```python
from build123d import *

# Parameters (mm, degrees)
SKETCH1_R           = 14.2875
SKETCH1_R_2         = 9.5885
SKETCH1_R_3         = 3.175
SKETCH1_R_4         = 2.257278931
SKETCH1_R_5         = 2.521989484
SKETCH1_R_6         = 2.481468777
SKETCH1_R_7         = 3.567111366
BOSS_EXTRUDE1_DEPTH = 3.175
FILLET1_R           = 9.525
FILLET2_R           = 3.175
FILLET3_R           = 6.35


with BuildPart() as part:
    # Sketch1 → Boss-Extrude1 (new, symmetric)
    with BuildSketch(Plane.XY):
        with BuildLine():
            Line((-35.563882813, 47.798897166), (35.563882813, 47.798897166))
            Line((35.563882813, 47.798897166), (51.692882813, 47.798897166))
            Line((51.692882813, 47.798897166), (67.821882813, 31.669897166))
            Line((67.821882813, 31.669897166), (67.821882813, 15.540897166))
            ThreePointArc((67.821882813, 15.540897166), (62.208310766, -2.642969943), (47.321354383, -14.498084612))
            Line((47.321354383, -14.498084612), (7.26457678, -33.02))
            Line((7.26457678, -33.02), (-7.26457678, -33.02))
            Line((-7.26457678, -33.02), (-47.321354383, -14.498084612))
            ThreePointArc((-47.321354383, -14.498084612), (-62.208310766, -2.642969943), (-67.821882813, 15.540897166))
            Line((-67.821882813, 15.540897166), (-67.821882813, 31.669897166))
            Line((-67.821882813, 31.669897166), (-51.692882813, 47.798897166))
            Line((-51.692882813, 47.798897166), (-35.563882813, 47.798897166))
        make_face()
        Circle(SKETCH1_R, mode=Mode.SUBTRACT)
        with Locations((35.563882813, 15.540897166)):
            Circle(SKETCH1_R_2, mode=Mode.SUBTRACT)
        with Locations((-35.563882813, 15.540897166)):
            Circle(SKETCH1_R_2, mode=Mode.SUBTRACT)
        with Locations((-47.625, 0)):
            Circle(SKETCH1_R_3, mode=Mode.SUBTRACT)
        with Locations((47.625, 0)):
            Circle(SKETCH1_R_3, mode=Mode.SUBTRACT)
        with Locations((-35.563882813, 40.940897166)):
            Circle(SKETCH1_R_4, mode=Mode.SUBTRACT)
        with Locations((-35.563882813, -9.859102834)):
            Circle(SKETCH1_R_5, mode=Mode.SUBTRACT)
        with Locations((35.563882813, -9.859102834)):
            Circle(SKETCH1_R_6, mode=Mode.SUBTRACT)
        with Locations((35.563882813, 40.940897166)):
            Circle(SKETCH1_R_7, mode=Mode.SUBTRACT)
    extrude(amount=BOSS_EXTRUDE1_DEPTH, both=True)

    # Fillet1
    fillet1_edges = [part.edges().sort_by_distance(p)[0] for p in [
        (51.692882813, 47.798897166, 0),
        (-51.692882813, 47.798897166, 0),
    ]]
    fillet(fillet1_edges, radius=FILLET1_R)

    # Fillet2
    fillet2_edges = [part.edges().sort_by_distance(p)[0] for p in [
        (67.821882813, 31.669897166, 0),
        (-67.821882813, 31.669897166, 0),
    ]]
    fillet(fillet2_edges, radius=FILLET2_R)

    # Fillet3
    fillet3_edges = [part.edges().sort_by_distance(p)[0] for p in [
        (7.26457678, -33.02, 0),
        (-7.26457678, -33.02, 0),
    ]]
    fillet(fillet3_edges, radius=FILLET3_R)


solid = part.part
```
For this review, take the finished solid that the model builds, in its own axes (mm). Coordinates: 2 decimals unless noted, no trailing zeros. Order: outer loops, then holes, each group sorted by start corner. A loop starts at its lowest first (then second) coordinate and runs counter-clockwise, first axis right, second up. Notation, with made-up numbers: (55, 89.25) -> (100, 89.25) arc R23 cw to (100, 107.25) -> close; hole circle Ø2 at (-36, 16). An arc over 180 degrees is marked (long way). Use CSV: the item, a comma, the result in double quotes. Start each with the question number.
Item 1: Insertion check: pin 1 (4 mm diameter, centred on x = -35.56, y = 40.94, fed in from +Z); pin 2 (1 mm diameter, centred on x = -30.5, z = 1, fed in from -Y); pin 3 (2 mm diameter, centred on y = 6, z = 1.5, fed in from +X). Each pin has a flat end and moves straight along its axis. Give the tip position at first contact, or say it passes through.
Item 2: We need section B-B, the plane y = 22. Give the boundary of the cut face in (x, z) (3 decimals), then the cut area to 3 significant figures.
Item 3: Draft analysis for pull direction X (two halves, no side actions). For faces 1 (the face through (1, 17, 3.175)), 2 (the face through (67.822, 23, 0)), 3 (the face through (-44.597, 0.954, -0.044)), 4 (the face through (-37.42, -8.15, -0.04)), state which applies: pulls with the +X half, pulls with the -X half, needs draft (parallel to the pull), parting line crosses it, or undercut.
Item 4: We need section C-C, the plane z = -1.25. Give the number of separate pieces and of enclosed holes in the cut face, then the cut area to 3 significant figures.
Item 5: Wall thickness on probe 1 along X at (y, z) = (-8, 0); probe 2 along X at (y, z) = (16, 0.5); probe 3 along X at (y, z) = (24, -2): over which ranges is each line inside the solid? List them lowest first.
Item 6: We need section A-A, the plane x = 0. Give the boundary of the cut face in (y, z) (1 decimal), then the cut area to 3 significant figures.
Derived:
1,pin 1,"passes through"
1,pin 2,"stops at y = -22.51"
1,pin 3,"stops at x = 66.67"
2,outline,"(-67.822, -3.175) -> (-42.65, -3.175) -> (-42.65, 3.175) -> (-67.822, 3.175) -> close; (-28.477, -3.175) -> (28.477, -3.175) -> (28.477, 3.175) -> (-28.477, 3.175) -> close; (42.65, -3.175) -> (67.822, -3.175) -> (67.822, 3.175) -> (42.65, 3.175) -> close"
2,area,"681 mm^2"
3,face 1,"needs draft"
3,face 2,"pulls with the +X half"
3,face 3,"undercut"
3,face 4,"undercut"
4,separate pieces,"1"
4,enclosed holes,"9"
4,area,"7,480 mm^2"
5,probe 1,"x = -57.62 to -37.27, -33.86 to -11.84, 11.84 to 33.92, 37.21 to 57.62"
5,probe 2,"x = -67.82 to -45.14, -25.99 to 25.99, 45.14 to 67.82"
5,probe 3,"x = -67.82 to -40.08, -31.05 to 31.05, 40.08 to 67.82"
6,outline,"(-33, -3.2) -> (-14.3, -3.2) -> (-14.3, 3.2) -> (-33, 3.2) -> close; (14.3, -3.2) -> (47.8, -3.2) -> (47.8, 3.2) -> (14.3, 3.2) -> close"
6,area,"332 mm^2"
